from build123d import *

# Parameters (mm, degrees)
F1_DEPTH = 18
F2_R     = 4
F3_DEPTH = 37.001


with BuildPart() as f1:
    # F0 (on Top) → F1 (new body)
    with BuildSketch(Plane.XY):
        with BuildLine():
            Line((0, 140), (0, 0))
            Line((0, 0), (37, 0))
            Line((37, 0), (37, 40.427738))
            ThreePointArc((37, 40.427738), (17.5, 70.21448), (37, 100.001222))
            Line((37, 100.001222), (37, 122.08924))
            ThreePointArc((37, 122.08924), (34.006301, 130.967637), (36.497201, 140))
            Line((36.497201, 140), (0, 140))
        make_face()
    extrude(amount=F1_DEPTH)

    # F2 (on face) → F3 (cut, through all)
    with BuildSketch(Plane.YZ.offset(37)):
        with Locations((111, 9)):
            Circle(F2_R)
        with Locations((29, 9)):
            Circle(F2_R)
    extrude(amount=-F3_DEPTH, mode=Mode.SUBTRACT)


solid = f1.part
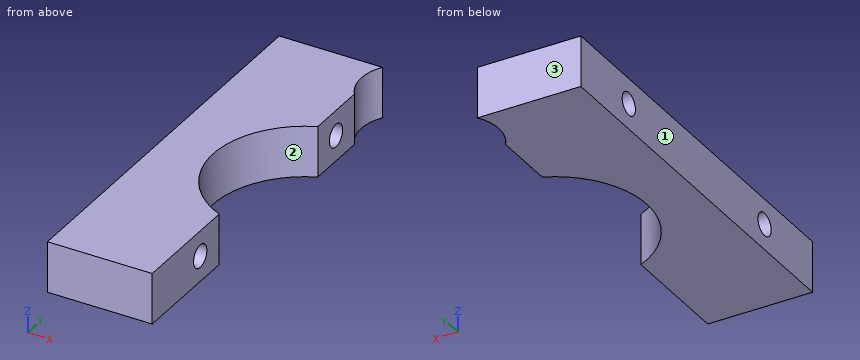
Work out the finished part from the listing and answer in its coordinate system (mm). Face numbers are marked on the shaded views. Round coordinates to 2 decimals unless told otherwise and drop trailing zeros. Write each loop counter-clockwise with the first axis right and the second up, starting at its lowest first coordinate (ties: lowest second). Pieces come first, ordered by that corner, then holes.
1) A cutting plane is placed at D-D (z = 14.75). Give the vertices of the cut face in (x, y), plus the area to 3 significant figures.
2) A cutting plane is placed at C-C (x = 24). Give the vertices of the cut face in (y, z).
3) Given pin 1 Ø7 at (y, z) = (29, 9) entering from -X, flat-ended and moving along its own axis, determine where the tip first touches the part or whether it passes through.
4) Straight lines are drawn through the part: line 1 (Z direction, x = 13.5, y = 111); line 2 (Y direction, x = 3, z = 10); line 3 (Y direction, x = 9, z = 12). For each, find the intervals that lie inside material, in ascending order.
5) A cutting plane is placed at B-B (z = 9). Give the vertices of the cut face in (x, y).
6) The mould has two halves that part along Y. Classify the marked faces 1, 2 and 3: pulls with the +Y half, pulls with the -Y half, needs draft (parallel to the pull), parting line crosses it, or undercut.
7) A cutting plane is placed at A-A (y = 111). Give the vertices of the cut face in (x, z).
Completed:
1. outline: (0, 0) - (37, 0) - (37, 40.43) arc R32.5 cw to (37, 100) - (37, 122.09) arc R16 cw to (36.5, 140) - (0, 140) - close
1. area: 4,300 mm2
2. outline: (0, 0) - (50.71, 0) - (50.71, 18) - (0, 18) - close; (89.71, 0) - (140, 0) - (140, 18) - (89.71, 18) - close; hole circle Ø8 at (29, 9); hole circle Ø8 at (111, 9)
3. pin 1: passes through
4. line 1: z = 0 to 5, 13 to 18
4. line 2: y = 0 to 25.13, 32.87 to 107.13, 114.87 to 140
4. line 3: y = 0 to 26.35, 31.65 to 108.35, 113.65 to 140
5. outline: (0, 0) - (37, 0) - (37, 25) - (0, 25) - close; (0, 33) - (37, 33) - (37, 40.43) arc R32.5 cw to (37, 100) - (37, 107) - (0, 107) - close; (0, 115) - (37, 115) - (37, 122.09) arc R16 cw to (36.5, 140) - (0, 140) - close
6. face 1: needs draft
6. face 2: undercut
6. face 3: pulls with the +Y half
7. outline: (0, 0) - (37, 0) - (37, 5) - (0, 5) - close; (0, 13) - (37, 13) - (37, 18) - (0, 18) - close
